from build123d import *

# Parameters (mm, degrees)
PAD_DEPTH = 15
FILLET_R  = 1


with BuildPart() as part:
    # Sketch → Pad (new body)
    with BuildSketch(Plane.XY):
        Polygon((0, 0), (0, 40), (51, 40), (51, 25), (26, 0), (26, 25), (10, 25), (10, 0), align=None)
    extrude(amount=PAD_DEPTH)

    # Fillet
    fillet_edges = [part.edges().sort_by_distance(p)[0] for p in [
        (5, 0, 15),
        (0, 0, 7.5),
        (10, 0, 7.5),
        (10, 12.5, 15),
        (18, 25, 15),
        (26, 12.5, 15),
        (38.5, 12.5, 15),
        (38.5, 12.5, 0),
        (26, 0, 7.5),
        (51, 25, 7.5),
        (0, 20, 15),
        (0, 20, 0),
        (0, 40, 7.5),
        (51, 32.5, 15),
        (18, 25, 0),
        (5, 0, 0),
        (10, 12.5, 0),
        (26, 12.5, 0),
        (25.5, 40, 0),
        (51, 32.5, 0),
        (51, 40, 7.5),
        (25.5, 40, 15),
    ]]
    fillet(fillet_edges, radius=FILLET_R)


solid = part.part
Here's how the part is built. I have some questions about the finished solid (model axes, mm). A direction names the side the tool comes from. Coordinates: 2 decimals unless noted, no trailing zeros. Loops run counter-clockwise (first coordinate to the right, second up) from the corner with the lowest first, then second, coordinate; pieces in that order, holes last. Notation, with made-up numbers: (58, 68.5) -> (106, 68.5) arc R26 ccw to (106, 98.5) -> close; hole circle Ø9 at (71.25, 57.5). An arc over 180 degrees is marked (long way). Use one line per item in the form item = value. Start each with the question number.
(1) If we section it at A-A (z = 8.25): Please give me the cut outline in (x, y).
(2) On a 3-axis mill with a long thin cutter (end or side, diameter ignored), from which of +Z, -Z, +X, -X, +Y, -Y can I reach the whole of each face in a straight line? I mean faces 4 (the face through (9.715, 13.325, 14.699)), 5 (the face through (18, 25, 7)), 6 (the face through (39, 13, 7)), 7 (the face through (26, 29, 15)), 8 (the face through (26.285, 14.372, 0.301)). Say none if no direction works.
(3) Please list where these lines run through material, in increasing order: line 1 along X through (y, z) = (24, 7.5); line 2 along X through (y, z) = (14, 9.5); line 3 along Y through (x, z) = (20.5, 4).
(4) Will these pins go through, and if not, where does the flat tip stop? pin 1 (6.5 mm diameter, centred on x = 21, z = 5.5, fed in from -Y); pin 2 (4 mm diameter, centred on y = 17.5, z = 10, fed in from +X); pin 3 (5 mm diameter, centred on x = 30, z = 2, fed in from -Y).
(5) We'd pull the mould along X, two halves only. Please class faces 1 (the face through (4.944, 0.285, 0.301)), 2 (the face through (17.874, 25.285, 0.301)), 3 (the face through (50.699, 39.715, 7.591)): pulls with the +X half, pulls with the -X half, needs draft (parallel to the pull), parting line crosses it, or undercut.
(6) If we section it at B-B (x = 11): Please give me the cut outline in (y, z).
Verdict:
q1.outline = (0, 1) arc R1 ccw to (1, 0) -> (9, 0) arc R1 ccw to (10, 1) -> (10, 25) -> (26, 25) -> (26, 2.41) arc R1 ccw to (27.71, 1.71) -> (50.71, 24.71) arc R1 ccw to (51, 25.41) -> (51, 39) arc R1 ccw to (50, 40) -> (1, 40) arc R1 ccw to (0, 39) -> close
q2.face_4 = +Z, -Y
q2.face_5 = +Z, -Z, -Y
q2.face_6 = +Z, -Z, +X, -Y
q2.face_7 = +Z, +X, -X, +Y, -Y
q2.face_8 = -Z, -Y
q3.line_1 = 0 to 10, 26 to 50
q3.line_2 = 0 to 10, 26 to 40
q3.line_3 = 25 to 40
q4.pin_1 = 25
q4.pin_2 = 45.5
q4.pin_3 = 1.55
q5.face_1 = needs draft
q5.face_2 = undercut
q5.face_3 = pulls with the +X half
q6.outline = (25, 1) arc R1 ccw to (26, 0) -> (39, 0) arc R1 ccw to (40, 1) -> (40, 14) arc R1 ccw to (39, 15) -> (26, 15) arc R1 ccw to (25, 14) -> close
